```python
from build123d import *

# Parameters (mm, degrees)
SKETCH3_R                   = 12.5
SKETCH3_R_2                 = 7.55
BOSS_EXTRUDE2_DEPTH         = 8.8
SKETCH4_W                   = 6.878404869
SKETCH4_H                   = 8
CUT_EXTRUDE2_DEPTH          = 8.8
SKETCH8_R                   = 10.34
CUT_EXTRUDE5_DEPTH          = 0.9
TAP_DRILL_FOR_M2X0_4_TAP1_D = 1.6
CUT_EXTRUDE6_DEPTH          = 0.9
BOSS_EXTRUDE4_DEPTH         = 2
FILLET2_R                   = 1
FILLET3_R                   = 1
M2_5_CLEARANCE_HOLE1_D      = 2.9
FILLET4_R                   = 1
FILLET5_R                   = 1


with BuildPart() as part:
    # Sketch3 → Boss-Extrude2 (new body)
    with BuildSketch(Plane(origin=(0, 0, 0), x_dir=(1, 0, 0), z_dir=(0, 1, 0))):
        with Locations(Location((0, 0, 0), (0, 0, 270))):
            Circle(SKETCH3_R)
        with Locations(Location((0, 0, 0), (0, 0, 270))):
            Circle(SKETCH3_R_2, mode=Mode.SUBTRACT)
    extrude(amount=BOSS_EXTRUDE2_DEPTH)

    # Sketch4 → Cut-Extrude2 (cut)
    with BuildSketch(Plane(origin=(0, 8.8, 0), x_dir=(1, 0, 0), z_dir=(0, 1, 0))):
        with Locations((9.842521887, 0)):
            Rectangle(SKETCH4_W, SKETCH4_H)
    extrude(amount=-CUT_EXTRUDE2_DEPTH, mode=Mode.SUBTRACT)

    # Sketch8 → Cut-Extrude5 (cut)
    with BuildSketch(Plane(origin=(0, 8.8, 0), x_dir=(1, 0, 0), z_dir=(0, 1, 0))):
        Circle(SKETCH8_R)
    extrude(amount=-CUT_EXTRUDE5_DEPTH, mode=Mode.SUBTRACT)

    # Tap Drill for M2x0.4 Tap1 (through all)
    with Locations(Plane(origin=(6.72, 8.8, 6.715027923), x_dir=(0, 0, 1), z_dir=(0, 1, 0))):
        with Locations((0, 0), (0.004972077, -13.435027923), (-13.435027923, -13.435027923), (-13.430055846, 0)):
            Hole(TAP_DRILL_FOR_M2X0_4_TAP1_D / 2)

    # Sketch11 → Cut-Extrude6 (cut)
    with BuildSketch(Plane(origin=(0, 8.8, 0), x_dir=(1, 0, 0), z_dir=(0, 1, 0))):
        with BuildLine():
            Line((8.889256072, 5.281735177), (5.288313257, 8.885344275))
            ThreePointArc((5.288313257, 8.885344275), (8.559157895, 8.552825038), (8.889256072, 5.281735177))
        make_face()
        with BuildLine():
            Line((8.889256072, -5.281735177), (5.288313257, -8.885344275))
            ThreePointArc((5.288313257, -8.885344275), (8.559157895, -8.552825038), (8.889256072, -5.281735177))
        make_face()
        with BuildLine():
            Line((-5.281735177, -8.889256072), (-8.885344275, -5.288313257))
            ThreePointArc((-8.885344275, -5.288313257), (-8.552825038, -8.559157895), (-5.281735177, -8.889256072))
        make_face()
        with BuildLine():
            Line((-5.281735177, 8.889256072), (-8.885344275, 5.288313257))
            ThreePointArc((-8.885344275, 5.288313257), (-8.552825038, 8.559157895), (-5.281735177, 8.889256072))
        make_face()
    extrude(amount=-CUT_EXTRUDE6_DEPTH, mode=Mode.SUBTRACT)

    # Sketch12 → Boss-Extrude4 (add)
    with BuildSketch(Plane.XZ):
        with BuildLine():
            Line((23.125, -23.125), (-23.125, -23.125))
            Line((-23.125, -23.125), (-23.125, 23.125))
            Line((-23.125, 23.125), (23.125, 23.125))
            Line((23.125, 23.125), (23.125, 4))
            Line((23.125, 4), (6.403319452, 4))
            ThreePointArc((6.403319452, 4), (-7.55, 0), (6.403319452, -4))
            Line((6.403319452, -4), (23.125, -4))
            Line((23.125, -4), (23.125, -23.125))
        make_face()
    extrude(amount=-BOSS_EXTRUDE4_DEPTH)

    # Fillet2
    fillet2_edges = [part.edges().sort_by_distance(p)[0] for p in [
        (0, 0, 23.125),
        (-23.125, 0, 0),
    ]]
    fillet(fillet2_edges, radius=FILLET2_R)

    # Fillet3
    # the kernel refuses this fillet: 1 mm, written as the material it takes off along each edge
    with BuildSketch(Plane(origin=(-22.125, 1, 22.125), x_dir=(0, 0, 1), z_dir=(-1, 0, 0))) as fillet3_piece_1_section:
        Polygon((0, 0), (FILLET3_R, 0), (FILLET3_R, -FILLET3_R), (0, -FILLET3_R), align=None)
    fillet3_piece_1 = extrude(amount=FILLET3_R, mode=Mode.PRIVATE)
    fillet3_piece_1 = fillet3_piece_1 - Plane(origin=(-22.125, 1, 22.125), x_dir=(0, 0.7071067811865475, -0.7071067811865475), z_dir=(-1, 0, 0)) * Sphere(FILLET3_R, mode=Mode.PRIVATE)
    add(fillet3_piece_1, mode=Mode.SUBTRACT)
    with BuildSketch(Plane(origin=(-23.125, 1, 23.125), x_dir=(0, 0, -1), z_dir=(0, 1, 0))) as fillet3_piece_2:
        with BuildLine():
            CenterArc((FILLET3_R, -FILLET3_R), FILLET3_R, 90, 90)
            Line((0, -FILLET3_R), (0, 0))
            Line((0, 0), (FILLET3_R, 0))
        make_face()
    extrude(amount=3.5, mode=Mode.SUBTRACT)

    # M2.5 Clearance Hole1 (through all)
    with Locations(Plane(origin=(18.3989, 0, 18.3989), x_dir=(0, 0, -1), z_dir=(0, -1, 0))):
        with Locations((0, 0), (36.7978, 0), (36.7978, -36.7978), (0, -36.7978)):
            Hole(M2_5_CLEARANCE_HOLE1_D / 2)

    # Fillet4
    fillet4_edges = [part.edges().sort_by_distance(p)[0] for p in [
        (23.125, 0, 13.0625),
        (23.125, 0, -13.5625),
        (-23.125, 1.5, -23.125),
        (23.125, 1.5, 23.125),
        (0.5, 0, -23.125),
        (-22.832106781, 0.292893219, -23.125),
        (23.125, 0.292893219, 22.832106781),
    ]]
    fillet(fillet4_edges, radius=FILLET4_R)

    # Fillet5
    # the kernel refuses this fillet: 1 mm, written as the material it takes off along each edge
    with BuildSketch(Plane(origin=(22.125, 1, -22.125), x_dir=(1, 0, 0), z_dir=(0, 0, -1))) as fillet5_piece_1_section:
        Polygon((0, 0), (FILLET5_R, 0), (FILLET5_R, FILLET5_R), (0, FILLET5_R), align=None)
    fillet5_piece_1 = extrude(amount=FILLET5_R, mode=Mode.PRIVATE)
    fillet5_piece_1 = fillet5_piece_1 - Plane(origin=(22.125, 1, -22.125), x_dir=(-0.7071067811865475, 0.7071067811865475, 0), z_dir=(0, 0, -1)) * Sphere(FILLET5_R, mode=Mode.PRIVATE)
    add(fillet5_piece_1, mode=Mode.SUBTRACT)
    with BuildSketch(Plane(origin=(23.125, 1, -23.125), x_dir=(-1, 0, 0), z_dir=(0, 1, 0))) as fillet5_piece_2:
        with BuildLine():
            CenterArc((FILLET5_R, FILLET5_R), FILLET5_R, 180, 90)
            Line((0, FILLET5_R), (0, 0))
            Line((0, 0), (FILLET5_R, 0))
        make_face()
    extrude(amount=3.5, mode=Mode.SUBTRACT)


solid = part.part
```
Could you check a few things on this model? Use its own coordinates, in mm. A direction names the side the tool comes from. Round coordinates to 2 decimals unless told otherwise and drop trailing zeros. Loops run counter-clockwise (first coordinate to the right, second up) from the corner with the lowest first, then second, coordinate; pieces in that order, holes last.
Q1. I want a section at B-B (z = 0). Write out the boundary of the cut face in (x, y) (3 decimals).
Q2. For P1, Ø1.8, axis at x = 6.5, z = -7, coming from the +Y side; P2, Ø5, axis at x = 13.5, z = 16.5, coming from the +Y side; P3, Ø1, axis at y = 3.5, z = 6.5, coming from the -X side; P4, Ø2.5, axis at x = -18.4, z = 18.4, coming from the -Y side, each with a flat end and sliding along its axis, tell me the tip position at first contact or that it passes through.
Q3. On a 3-axis mill with a long thin cutter (end or side, diameter ignored), from which of +Z, -Z, +X, -X, +Y, -Y can I reach the whole of each face in a straight line? I mean faces 1 (the flat face through (11, 3, -4)), 2 (the flat face through (23.125, 1.5, -12.9)), 3 (the cylindrical face through (8.52, 8.36, -8.59)). Say none if no direction works.
Q4. Thinking about a two-plate mould opening in Z: for faces 4 (the cylindrical face through (-0.31, 0.3, -22.84)), 5 (the cylindrical face through (22.824, 0.285, 12.936)), 6 (the flat face through (-8, 7.9, 0)), which applies, pulls with the +Z half, pulls with the -Z half, needs draft (parallel to the pull), parting line crosses it, or undercut?
Q5. I want a section at C-C (y = 6.75). Write out the boundary of the cut face in (x, z).
Q6. I want a section at D-D (z = -6.72). Write out the boundary of the cut face in (x, y) (3 decimals).
Q7. Please list where these lines run through material, in increasing order: L1, parallel to Z at x = 0, y = 3.25; L2, parallel to Z at x = 20.5, y = 1 (3 decimals); L3, parallel to Y at x = 4, z = -13.5.
Q8. I want a section at A-A (x = 0). Write out the boundary of the cut face in (y, z) (3 decimals), and give its area (3 significant figures).
Answer below:
1. outline: (-23.125, 1) arc R1 ccw to (-22.125, 0) - (-7.55, 0) - (-7.55, 7.9) - (-10.34, 7.9) - (-10.34, 8.8) - (-12.5, 8.8) - (-12.5, 2) - (-23.125, 2) - close
2. P1: stops at y = 7.9
2. P2: stops at y = 2
2. P3: stops at x = -10.97
2. P4: passes through
3. face 1: +X, +Y, -Y
3. face 2: +Z, -Z, +X, +Y, -Y
3. face 3: +Y
4. face 4: pulls with the -Z half
4. face 5: needs draft
4. face 6: undercut
5. outline: (6.4, -4) arc R7.55 cw (long way) to (6.4, 4) - (11.84, 4) arc R12.5 ccw (long way) to (11.84, -4) - close; hole circle Ø1.6 at (-6.72, -6.72); hole circle Ø1.6 at (-6.72, 6.72); hole circle Ø1.6 at (6.72, -6.72); hole circle Ø1.6 at (6.72, 6.72)
6. outline: (-23.125, 1) arc R1 ccw to (-22.125, 0) - (-3.442, 0) - (-3.442, 7.9) - (-5.915, 7.9) - (-5.915, 2) - (-7.515, 2) - (-7.515, 7.9) - (-9.315, 7.9) - (-9.315, 8.8) - (-10.54, 8.8) - (-10.54, 2) - (-23.125, 2) - close; (3.442, 0) - (22.125, 0) arc R1 ccw to (23.125, 1) - (23.125, 2) - (10.54, 2) - (10.54, 8.8) - (9.32, 8.8) - (9.32, 7.9) - (7.52, 7.9) - (7.52, 2) - (5.92, 2) - (5.92, 7.9) - (3.442, 7.9) - close
7. L1: z = -12.5 to -7.55, 7.55 to 12.5
7. L2: z = -23.125 to -4, 4 to 23.125
7. L3: y = 0 to 2
8. outline: (0, -22.125) arc R1 ccw to (1, -23.125) - (2, -23.125) - (2, -12.5) - (8.8, -12.5) - (8.8, -10.34) - (7.9, -10.34) - (7.9, -7.55) - (0, -7.55) - close; (0, 7.55) - (7.9, 7.55) - (7.9, 10.34) - (8.8, 10.34) - (8.8, 12.5) - (2, 12.5) - (2, 23.125) - (1, 23.125) arc R1 ccw to (0, 22.125) - close
8. area: 124 mm2
